from build123d import *

# Parameters (mm, degrees)
F0_W     = 35.2719388902
F0_H     = 81.6293433309
F1_DEPTH = 25
F2_R     = 12.7443419247
F3_DEPTH = 25
F4_DEPTH = 50
F5_SIZE  = 5
F6_SIZE  = 2
F7_SIZE  = 10


with BuildPart() as f1:
    # F0 (on Top) → F1 (new body)
    with BuildSketch(Plane.XY):
        Rectangle(F0_W, F0_H)
    extrude(amount=F1_DEPTH)

    # F2 (on Top) → F3 (cut)
    with BuildSketch(Plane.XY):
        with Locations((0, 25.8420929313)):
            Circle(F2_R)
    extrude(amount=F3_DEPTH, mode=Mode.SUBTRACT)

    # F4 (add): a face of the model
    f4_faces = [f1.faces().sort_by_distance(p)[0] for p in [
        (0, -40.8146716654, 12.5),
    ]]
    extrude(f4_faces, amount=F4_DEPTH)

    # F5
    f5_edges = [f1.edges().sort_by_distance(p)[0] for p in [
        (-17.635969, 40.814672, 12.5),
        (17.635969, 40.814672, 12.5),
    ]]
    chamfer(f5_edges, length=F5_SIZE)

    # F6
    f6_edges = [f1.edges().sort_by_distance(p)[0] for p in [
        (17.635969, -27.5, 25),
        (-17.635969, -27.5, 25),
        (17.635969, -27.5, 0),
        (-17.635969, -27.5, 0),
    ]]
    chamfer(f6_edges, length=F6_SIZE)

    # F7 (call 1 of 4: OpenCascade refuses the feature's edges together)
    f7_edges = [f1.edges().sort_by_distance(p)[0] for p in [
        (0, -90.814672, 25),
    ]]
    chamfer(f7_edges, length=F7_SIZE)

    # F7#2 (call 2 of 4)
    f7_2_edges = [f1.edges().sort_by_distance(p)[0] for p in [
        (17.635969, -90.814672, 12.5),
    ]]
    chamfer(f7_2_edges, length=F7_SIZE)

    # F7#3 (call 3 of 4)
    f7_3_edges = [f1.edges().sort_by_distance(p)[0] for p in [
        (0, -90.814672, 0),
    ]]
    chamfer(f7_3_edges, length=F7_SIZE)

    # F7#4 (call 4 of 4)
    f7_4_edges = [f1.edges().sort_by_distance(p)[0] for p in [
        (-17.635969, -90.814672, 12.5),
    ]]
    chamfer(f7_4_edges, length=F7_SIZE)


solid = f1.part
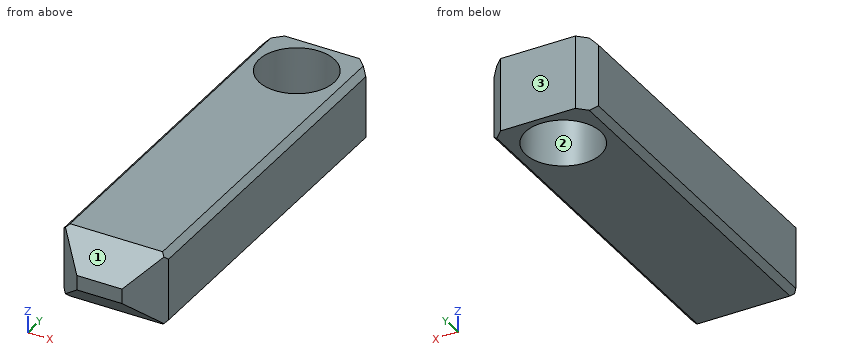
Geometry check sheet. Reference: the model listing, model coordinates, mm. Face numbers are marked on the shaded views. Give positions to 0.01 mm unless a question says otherwise; leave off trailing zeros. Loops run counter-clockwise (first coordinate to the right, second up) from the corner with the lowest first, then second, coordinate; pieces in that order, holes last. Notation, with made-up numbers: M 3.5,7 L 50.5,7 A8 cw 50.5,12 Z; hole C -16,16.5 d11. An arc over 180 degrees is marked long. Answer as a JSON object with one key per item and string values. Group by question number.
Item 1: Sectioned sample at D-D on z = 13. Record the boundary of the cut face in (x, y), plus the area to 3 significant figures.
Item 2: Material ranges on L1, parallel to Y at x = 6.5, z = 23.5; L2, parallel to Y at x = -8.5, z = 23; L3, parallel to X at y = -36, z = 1, recorded low to high.
Item 3: Sectioned sample at C-C on x = 5. Record the boundary of the cut face in (y, z), plus the area to 3 significant figures.
Item 4: Gauge pin test, flat end, axial feed: pin 1 (2 mm diameter, centred on x = 1.5, z = 4.5, fed in from -Y). Record the tip position at first contact, or that the pin passes through.
Item 5: Sectioned sample at B-B on z = 4. Record the boundary of the cut face in (x, y).
Item 6: Sectioned sample at A-A on x = 0. Record the boundary of the cut face in (y, z).
Item 7: Mould release check, pull along Y, two halves, no side actions. Record for the marked faces 1, 2 and 3: pulls with the +Y half, pulls with the -Y half, needs draft (parallel to the pull), parting line crosses it, or undercut.
Findings below:
{
 "1": {"outline": "M -17.64,-80.81 L -7.64,-90.81 L 7.64,-90.81 L 17.64,-80.81 L 17.64,35.81 L 12.64,40.81 L -12.64,40.81 L -17.64,35.81 Z; hole C 0,25.84 d25.49", "area": "4,010 mm2"},
 "2": {"L1": "-82.31 to 14.88, 36.8 to 40.81", "L2": "-82.81 to 16.35, 35.34 to 40.81", "L3": "-16.64 to 16.64"},
 "3": {"outline": "M -90.81,10 L -80.81,0 L 14.12,0 L 14.12,25 L -80.81,25 L -90.81,15 Z; M 37.56,0 L 40.81,0 L 40.81,25 L 37.56,25 Z", "area": "2,600 mm2"},
 "4": {"pin 1": "y = -86.31"},
 "5": {"outline": "M -17.64,-80.81 L -13.64,-84.81 L 13.64,-84.81 L 17.64,-80.81 L 17.64,35.81 L 12.64,40.81 L -12.64,40.81 L -17.64,35.81 Z; hole C 0,25.84 d25.49"},
 "6": {"outline": "M -90.81,10 L -80.81,0 L 13.1,0 L 13.1,25 L -80.81,25 L -90.81,15 Z; M 38.59,0 L 40.81,0 L 40.81,25 L 38.59,25 Z"},
 "7": {"face 1": "pulls with the -Y half", "face 2": "undercut", "face 3": "pulls with the +Y half"}
}
